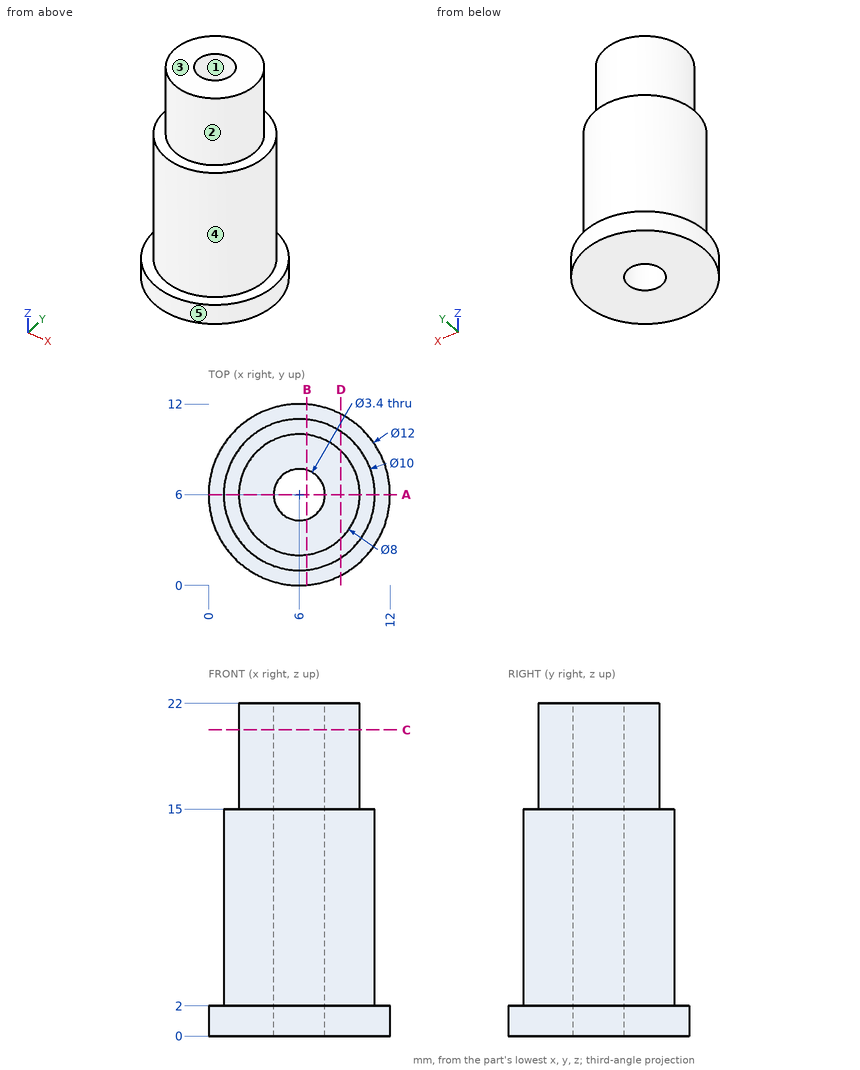
Design review of the part shown in the three views and the two pictorial views. Dimensions are in mm from the part's minimum x, y and z. A direction names the side the tool comes from. Round coordinates to 2 decimals unless told otherwise and drop trailing zeros. Loops run counter-clockwise (first coordinate to the right, second up) from the corner with the lowest first, then second, coordinate; pieces in that order, holes last. Notation, with made-up numbers: M 84.25,55 L 106.25,55 A21 ccw 106.25,74 Z; hole C 18,11.5 d9. An arc over 180 degrees is marked long. Answer as a JSON object with one key per item and string values.
Item 1: We need section A-A on y = 6. Give the boundary of the cut face in (x, z), and give its area (3 significant figures).
Answer sheet:
{"outline": "M 0,0 L 4.3,0 L 4.3,22 L 2,22 L 2,15 L 1,15 L 1,2 L 0,2 Z; M 7.7,0 L 12,0 L 12,2 L 11,2 L 11,15 L 10,15 L 10,22 L 7.7,22 Z", "area": "135 mm^2"}
Item 2: We need section C-C on z = 20.25. Give the boundary of the cut face in (x, y), and give its area (3 significant figures).
Answer sheet:
{"outline": "C 6,6 d8; hole C 6,6 d3.4", "area": "41.2 mm^2"}
Item 3: Machinability: for the marked faces 4 and 5, which of the approach directions +Z, -Z, +X, -X, +Y, -Y give a long, thin tool a straight path to every point of the face, cutting with its end or side? Answer none if there is none.
Answer sheet:
{"face 4": "+Z", "face 5": "+Z, -Z"}
Item 4: Clearance check with flat-ended pins moving along their axes: P1, Ø4.5, axis at x = 6, y = 6, coming from the -Z side; P2, Ø1.5, axis at x = 5.5, z = 9, coming from the +Y side; P3, Ø1, axis at x = 5.5, y = 5.5, coming from the -Z side; P4, Ø3, axis at y = 10.5, z = 6, coming from the +X side. State where each tip first meets the part, or that it passes through.
Answer sheet:
{"P1": "stops at z = 0", "P2": "stops at y = 11", "P3": "passes through", "P4": "stops at x = 10"}
Item 5: We need section D-D on x = 8.75. Give the boundary of the cut face in (y, z), and give its area (3 significant figures).
Answer sheet:
{"outline": "M 0.67,0 L 11.33,0 L 11.33,2 L 10.18,2 L 10.18,15 L 8.9,15 L 8.9,22 L 3.1,22 L 3.1,15 L 1.82,15 L 1.82,2 L 0.67,2 Z", "area": "171 mm^2"}
Item 6: Wall thickness on L1, parallel to Y at x = 6, z = 9.5; L2, parallel to Z at x = 1.5, y = 6.5; L3, parallel to Y at x = 6, z = 15.5: over which ranges is each line inside the solid? List them lowest first. Write a range as from..to.
Answer sheet:
{"L1": "y = 1..4.3, 7.7..11", "L2": "z = 0..15", "L3": "y = 2..4.3, 7.7..10"}
Item 7: The part is to be moulded in two halves that separate along Y. For the marked faces 1, 2 and 3, say which applies: pulls with the +Y half, pulls with the -Y half, needs draft (parallel to the pull), parting line crosses it, or undercut.
Answer sheet:
{"face 1": "undercut", "face 2": "parting line crosses it", "face 3": "needs draft"}
Item 8: We need section B-B on x = 6.5. Give the boundary of the cut face in (y, z), and give its area (3 significant figures).
Answer sheet:
{"outline": "M 0.02,0 L 4.38,0 L 4.38,22 L 2.03,22 L 2.03,15 L 1.03,15 L 1.03,2 L 0.02,2 Z; M 7.62,0 L 11.98,0 L 11.98,2 L 10.97,2 L 10.97,15 L 9.97,15 L 9.97,22 L 7.62,22 Z", "area": "137 mm^2"}
